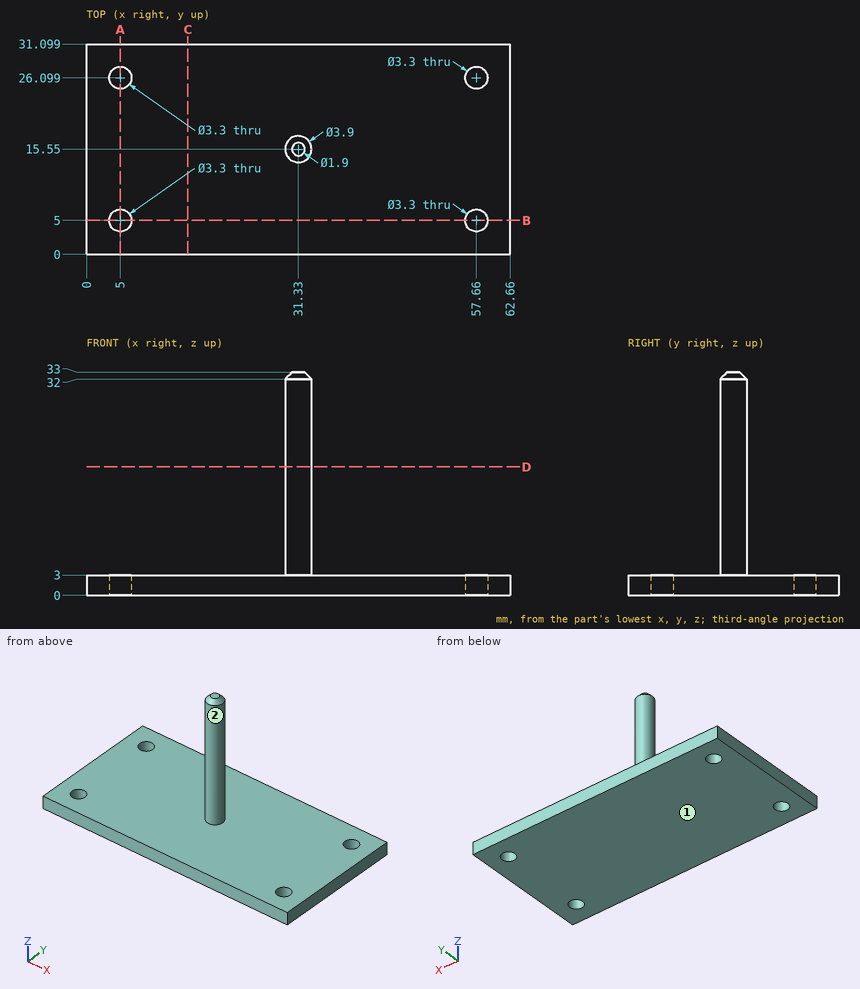
Can you work these out from the drawing? Everything is in mm from the part's minimum corner. A direction names the side the tool comes from. Coordinates: 2 decimals unless noted, no trailing zeros. Order: outer loops, then holes, each group sorted by start corner. A loop starts at its lowest first (then second) coordinate and runs counter-clockwise, first axis right, second up. Notation, with made-up numbers: M 78,7 L 98,7 A6 ccw 98,15 Z; hole C 28,12.25 d11. An arc over 180 degrees is marked long. Answer as CSV lines item,"result". Start each with the question number.
1. I need wall thicknesses on line 1 (Y direction, x = 5, z = 2.05); line 2 (Z direction, x = 38.5, y = 10.5); line 3 (X direction, y = 6, z = 2). Which ranges of each line are inside material? Lowest first, please. Write a range as [from, to].
2. I want a section at B-B, the plane y = 5. Write out the boundary of the cut face in (x, z).
3. For pin 1 (5 mm diameter, centred on x = 43.5, y = 25.5, fed in from +Z); pin 2 (4 mm diameter, centred on y = 12, z = 27.5, fed in from +X) (1 decimal), each with a flat end and sliding along its axis, tell me the tip position at first contact or that it passes through.
4. I want a section at C-C, the plane x = 15. Write out the boundary of the cut face in (y, z).
5. I want a section at D-D, the plane z = 19. Write out the boundary of the cut face in (x, y).
6. I want a section at A-A, the plane x = 5. Write out the boundary of the cut face in (y, z).
7. On a 3-axis mill with a long thin cutter (end or side, diameter ignored), from which of +Z, -Z, +X, -X, +Y, -Y can I reach the whole of each face in a straight line? I mean the marked faces 1 and 2. Say none if no direction works.
Recorded:
1,line 1,"y = [0, 3.35], [6.65, 24.45], [27.75, 31.1]"
1,line 2,"z = [0, 3]"
1,line 3,"x = [0, 3.69], [6.31, 56.35], [58.97, 62.66]"
2,outline,"M 0,0 L 3.35,0 L 3.35,3 L 0,3 Z; M 6.65,0 L 56.01,0 L 56.01,3 L 6.65,3 Z; M 59.31,0 L 62.66,0 L 62.66,3 L 59.31,3 Z"
3,pin 1,"stops at z = 3"
3,pin 2,"stops at x = 32.5"
4,outline,"M 0,0 L 31.1,0 L 31.1,3 L 0,3 Z"
5,outline,"C 31.33,15.55 d3.9"
6,outline,"M 0,0 L 3.35,0 L 3.35,3 L 0,3 Z; M 6.65,0 L 24.45,0 L 24.45,3 L 6.65,3 Z; M 27.75,0 L 31.1,0 L 31.1,3 L 27.75,3 Z"
7,face 1,"-Z, +X, -X, +Y, -Y"
7,face 2,"+Z"
